Geometry: see drawing. Coordinates: mm, zero at the bounding-box minimum. Coordinates: 2 decimals unless noted, no trailing zeros. Loops run counter-clockwise (first coordinate to the right, second up) from the corner with the lowest first, then second, coordinate; pieces in that order, holes last. Notation, with made-up numbers: (22.5, 4) - (73.5, 4) arc R29 cw to (73.5, 31) - close; hole circle Ø4 at (76.5, 69.5). An arc over 180 degrees is marked (long way). Use one line per item in the form item = value.
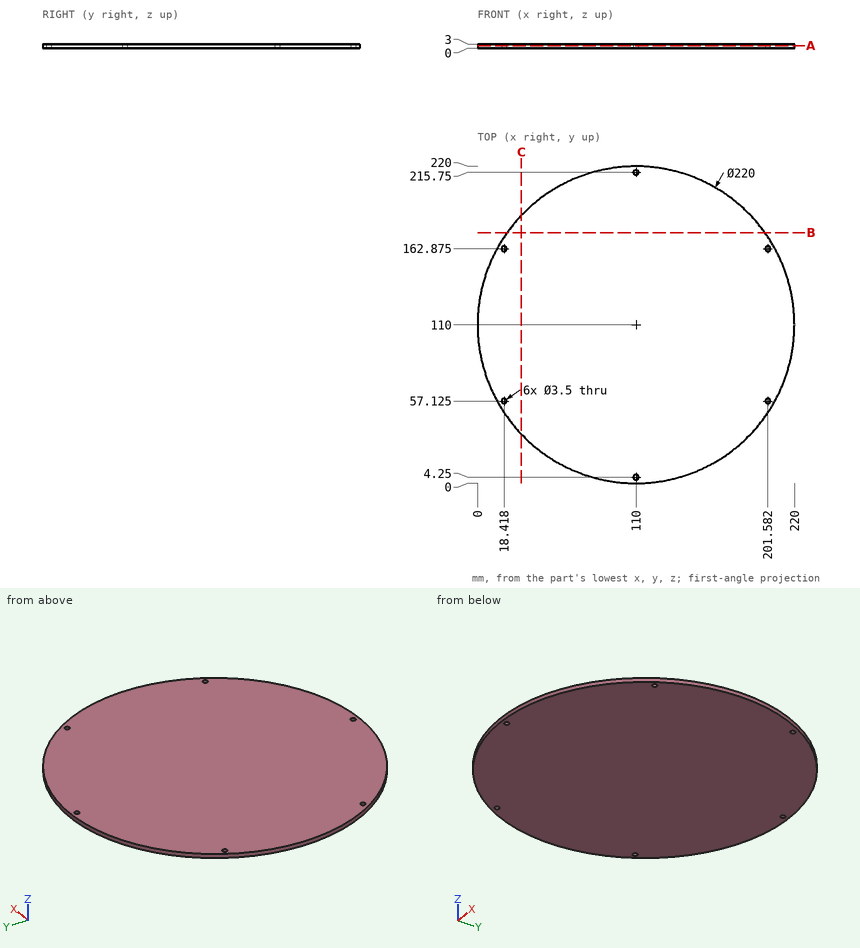
Q1. Ray query, line 1 along Y through (x, z) = (110, 1.65); line 2 along Y through (x, z) = (15, 1.8); line 3 along Y through (x, z) = (40.5, 2.9). Return the intervals inside material, ascending. Write a range as [from, to].
Check values:
line_1 = [0, 2.5], [6, 214], [217.5, 220]
line_2 = [54.55, 165.45]
line_3 = [24.74, 195.26]
Q2. Cut plane B-B, the plane y = 174. Return loops of the section in (x, z) (3 decimals).
Check values:
outline = (20.535, 0) - (199.465, 0) - (199.465, 3) - (20.535, 3) - close
Q3. Cut plane C-C, the plane x = 30.5. Return loops of the section in (y, z) (1 decimal).
Check values:
outline = (34, 0) - (186, 0) - (186, 3) - (34, 3) - close
Q4. First-contact query: P1, Ø3, axis at x = 201.58, y = 57.12, coming from the +Z side; P2, Ø1, axis at y = 24, z = 2, coming from the -X side; P3, Ø1, axis at x = 193.5, z = 1.5, coming from the +Y side. Flat tips, straight axial feed; report the tip coordinate or a pass-through.
Check values:
P1 = through
P2 = 40.79
P3 = 182.19
Q5. Cut plane A-A, the plane z = 1.8. Give the number of separate pieces and of enclosed holes in the cut face, then the cut area to 3 significant figures.
Check values:
separate_pieces = 1
enclosed_holes = 6
area = 38,000 mm²
